from build123d import *

# Parameters (mm, degrees)
F1_DEPTH = 63.5
F2_DEPTH = 38.1
F3_DEPTH = 7.9375
F0_W     = 25.4
F0_H     = 19.05
F5_R     = 6.35


with BuildPart() as f1:
    # F0 (on Front) → F1 (new body, symmetric)
    with BuildSketch(Plane.XZ):
        Polygon((-41.275, -9.525), (41.275, -9.525), (41.275, 9.525), (22.225, 9.525), (-41.275, 9.525), align=None)
    extrude(amount=F1_DEPTH, both=True)

    # F0 (on Front) → F2 (join, symmetric)
    with BuildSketch(Plane.XZ):
        with BuildLine():
            Line((22.225, 9.525), (41.275, 9.525))
            Line((41.275, 9.525), (41.275, 33.4762879004))
            ThreePointArc((41.275, 33.4762879004), (44.5168460124, 40.6164151559), (52.0260985597, 42.8752))
            Line((52.0260985597, 42.8752), (65.8047579605, 42.8752))
            Line((65.8047579605, 42.8752), (65.8047579605, 61.9252))
            Line((65.8047579605, 61.9252), (52.9601850462, 61.9252))
            ThreePointArc((52.9601850462, 61.9252), (31.3762728586, 54.4166329279), (22.225, 33.4762879004))
            Line((22.225, 33.4762879004), (22.225, 9.525))
        make_face()
    extrude(amount=F2_DEPTH, both=True)

    # F0 (on Front) → F3 (join, symmetric)
    with BuildSketch(Plane.XZ):
        with BuildLine():
            add(Edge.make_bspline(
                [(-41.275, 9.525), (-33.4530882537, 46.4520864189), (4.1069700383, 68.8830763102), (65.8047579605, 66.675)],
                knots=[0, 0, 0, 0, 121.3762623616, 121.3762623616, 121.3762623616, 121.3762623616], degree=3))
            Line((-41.275, 9.525), (22.225, 9.525))
            Line((22.225, 9.525), (22.225, 33.4762879004))
            ThreePointArc((22.225, 33.4762879004), (31.3762728586, 54.4166329279), (52.9601850462, 61.9252))
            Line((52.9601850462, 61.9252), (65.8047579605, 61.9252))
            Line((65.8047579605, 61.9252), (65.8047579605, 66.675))
        make_face()
    extrude(amount=F3_DEPTH, both=True)

    # F0 (on Front) → F4 (revolve)
    with BuildSketch(Plane.XZ):
        with Locations((78.5047579605, 52.4002)):
            Rectangle(F0_W, F0_H)
    revolve(axis=Axis((65.8047579605, 0, 52.3875), (0, 0, 1)))

    # F5
    f5_edges = [f1.edges().sort_by_distance(p)[0] for p in [
        (41.275, -63.5, 0),
        (41.275, 63.5, 0),
        (-41.275, 63.5, 0),
        (-41.275, -63.5, 0),
    ]]
    fillet(f5_edges, radius=F5_R)


solid = f1.part
The model under review builds one solid part; all positions refer to its coordinate system, in mm. A direction names the side the tool comes from. Round coordinates to 2 decimals unless told otherwise and drop trailing zeros. Order: outer loops, then holes, each group sorted by start corner. A loop starts at its lowest first (then second) coordinate and runs counter-clockwise, first axis right, second up. Notation, with made-up numbers: (31.5, 74.25) -> (75.5, 74.25) arc R5 ccw to (75.5, 81.25) -> close; hole circle Ø2 at (34.5, 55.25). An arc over 180 degrees is marked (long way). Return JSON: item names as keys, results as strings.
1. For L1, parallel to Y at x = 28, z = 12; L2, parallel to Y at x = -10, z = 30.5; L3, parallel to Z at x = 20, y = -36 (3 decimals), list the stretches that pass through material, from the lowest coordinate up. Write a range as [from, to].
Answer block:
{"L1": "y = [-38.1, 38.1]", "L2": "y = [-7.94, 7.94]", "L3": "z = [-9.525, 9.525]"}
2. Insertion check: P1, Ø6.5, axis at y = -32, z = 47.5, coming from the +X side; P2, Ø3.5, axis at x = 47, y = 13.5, coming from the +Z side; P3, Ø16.5, axis at x = 6.5, y = -49.5, coming from the +Z side (3 decimals); P4, Ø2, axis at x = 42, y = -9.5, coming from the -Z side (3 decimals). Each pin has a flat end and moves straight along its axis. Give the tip position at first contact, or say it passes through.
Answer block:
{"P1": "stops at x = 65.8", "P2": "stops at z = 61.94", "P3": "stops at z = 9.525", "P4": "stops at z = -9.525"}
3. Take a section at A-A (y = 27). Write out the cut boundary in (x, z) (3 decimals), then the cut area to 3 significant figures.
Answer block:
{"outline": "(-41.275, -9.525) -> (41.275, -9.525) -> (41.275, 33.476) arc R9.484 cw to (52.026, 42.875) -> (65.805, 42.875) -> (65.805, 61.925) -> (52.96, 61.925) arc R28.534 ccw to (22.225, 33.476) -> (22.225, 9.525) -> (-41.275, 9.525) -> close", "area": "2,880 mm²"}
4. Take a section at C-C (y = -48.5). Write out the cut boundary in (x, z) (3 decimals).
Answer block:
{"outline": "(-41.275, -9.525) -> (41.275, -9.525) -> (41.275, 9.525) -> (-41.275, 9.525) -> close"}
5. For faces 1 (the face through (39, -38.1, 36)), 2 (the face through (43.069, 11.324, 61.546)), 3 (the face through (42.99, -11.16, 61.39)), 4 (the face through (65.805, 32, 52)), list the 3-axis set-ups (+Z, -Z, +X, -X, +Y, -Y) from which the entire face can be reached by the end or side of a thin tool; tool diameter is ignored.
Answer block:
{"face 1": "+Z, +X, -X, -Y", "face 2": "+Z, -X, +Y", "face 3": "+Z, -X, -Y", "face 4": "+Z, -Z, +X, +Y"}
6. Take a section at B-B (z = 5.5). Write out the cut boundary in (x, y) (3 decimals), then the cut area to 3 significant figures.
Answer block:
{"outline": "(-41.275, -57.15) arc R6.35 ccw to (-34.925, -63.5) -> (34.925, -63.5) arc R6.35 ccw to (41.275, -57.15) -> (41.275, 57.15) arc R6.35 ccw to (34.925, 63.5) -> (-34.925, 63.5) arc R6.35 ccw to (-41.275, 57.15) -> close", "area": "10,400 mm²"}
